from build123d import *

# Parameters (mm, degrees)
SKETCH1_W           = 590
SKETCH1_H           = 5
BOSS_EXTRUDE1_DEPTH = 9


with BuildPart() as part:
    # Sketch1 → Boss-Extrude1 (new body)
    with BuildSketch(Plane(origin=(0, 0, 0), x_dir=(1, 0, 0), z_dir=(0, 1, 0))):
        Polygon((0, 35), (0, 17.5), (30, 17.5), (25, 0), (270, 0), (265, 17.5), (295, 17.5), (295, 35), align=None)
        Polygon((590, 35), (295, 35), (295, 17.5), (325, 17.5), (320, 0), (565, 0), (560, 17.5), (590, 17.5), align=None)
        with Locations((295, 37.5)):
            Rectangle(SKETCH1_W, SKETCH1_H)
    extrude(amount=BOSS_EXTRUDE1_DEPTH)


solid = part.part
Geometry check sheet. Reference: the model listing, model coordinates, mm. A direction names the side the tool comes from. Round coordinates to 2 decimals unless told otherwise and drop trailing zeros. Loops run counter-clockwise (first coordinate to the right, second up) from the corner with the lowest first, then second, coordinate; pieces in that order, holes last.
Item 1: Cross-section at A-A on z = -5.5. Record the boundary of the cut face in (x, y).
Item 2: Thickness scan on line 1 (Z direction, x = 24.5, y = 2.75); line 2 (X direction, y = 3.25, z = -12); line 3 (X direction, y = 1.75, z = -16). Record the ranges inside material, lowest first.
Item 3: Mould release check, pull along X, two halves, no side actions. Record for faces 1 (the flat face through (295, 4, -17.5)), 2 (the flat face through (562.535, 4.437, -8.628)), 3 (the flat face through (291, 4, -40)), 4 (the flat face through (267.535, 4.437, -8.628)): pulls with the +X half, pulls with the -X half, needs draft (parallel to the pull), parting line crosses it, or undercut.
Item 4: Gauge pin test, flat end, axial feed: pin 1 (4.5 mm diameter, centred on x = 308.5, y = 5, fed in from +Z). Record the tip position at first contact, or that the pin passes through.
Item 5: Cross-section at C-C on x = 308.5. Record the boundary of the cut face in (y, z), then the cut area to 4 significant figures.
Item 6: Cross-section at B-B on y = 2.5. Record the boundary of the cut face in (x, z).
Item 7: Access from +Z, -Z, +X, -X, +Y, -Y to the whole of each face (thin tool, end or side, straight path). Record for faces 5 (the flat face through (27.535, 4.437, -8.872)), 6 (the flat face through (575, 4, -17.5)), 7 (the flat face through (291, 0, -20)).
Answer sheet:
1. outline: (26.57, 0) - (268.43, 0) - (268.43, 9) - (26.57, 9) - close; (321.57, 0) - (563.43, 0) - (563.43, 9) - (321.57, 9) - close
2. line 1: z = -40 to -17.5
2. line 2: x = 28.43 to 266.57, 323.43 to 561.57
2. line 3: x = 29.57 to 265.43, 324.57 to 560.43
3. face 1: undercut
3. face 2: pulls with the +X half
3. face 3: needs draft
3. face 4: undercut
4. pin 1: stops at z = -17.5
5. outline: (0, -40) - (9, -40) - (9, -17.5) - (0, -17.5) - close
5. area: 202.5 mm2
6. outline: (0, -40) - (590, -40) - (590, -17.5) - (560, -17.5) - (565, 0) - (320, 0) - (325, -17.5) - (265, -17.5) - (270, 0) - (25, 0) - (30, -17.5) - (0, -17.5) - close
7. face 5: -X, +Y, -Y
7. face 6: +X, +Y, -Y
7. face 7: +Z, -Z, +X, -X, -Y
